```python
from build123d import *

# Parameters (mm, degrees)
BOSS_EXTRUDE1_DEPTH = 25
SKETCH2_R           = 1.5
CUT_EXTRUDE1_DEPTH  = 8
CUT_EXTRUDE2_START  = -8
SKETCH3_R           = 1.5
CUT_EXTRUDE2_DEPTH  = 8


with BuildPart() as part:
    # Sketch1 → Boss-Extrude1 (new, symmetric)
    with BuildSketch(Plane(origin=(0, 0, 0), x_dir=(1, 0, 0), z_dir=(0, 1, 0))):
        Polygon((2.655811238, 0), (1.327905619, 2.3), (-1.327905619, 2.3), (-2.655811238, 0), (-1.327905619, -2.3), (1.327905619, -2.3), align=None)
    extrude(amount=BOSS_EXTRUDE1_DEPTH, both=True)

    # Sketch2 → Cut-Extrude1 (cut)
    with BuildSketch(Plane(origin=(0, 25, 0), x_dir=(1, 0, 0), z_dir=(0, 1, 0))):
        with Locations(Location((0, 0, 0), (0, 0, 270))):
            Circle(SKETCH2_R)
    extrude(amount=-CUT_EXTRUDE1_DEPTH, mode=Mode.SUBTRACT)

    # Sketch3 → Cut-Extrude2 (cut)
    with BuildSketch(Plane.XZ.offset(25).offset(CUT_EXTRUDE2_START)):
        with Locations(Location((0, 0, 0), (0, 0, 90))):
            Circle(SKETCH3_R)
    extrude(amount=CUT_EXTRUDE2_DEPTH, mode=Mode.SUBTRACT)


solid = part.part
```
Model file for the job. Use its own axes, mm. A direction names the side the tool comes from. Round coordinates to 2 decimals unless told otherwise and drop trailing zeros. Order: outer loops, then holes, each group sorted by start corner. A loop starts at its lowest first (then second) coordinate and runs counter-clockwise, first axis right, second up. Notation, with made-up numbers: (10.25, 59) -> (65.25, 59) arc R32 cw to (65.25, 94) -> close; hole circle Ø1 at (17, 53). An arc over 180 degrees is marked (long way). Use one line per item in the form item = value.
Item 1: Drill centre lines: line 1 (X direction, y = 21, z = 0); line 2 (Y direction, x = 0.45, z = -0.3); line 3 (X direction, y = 13, z = -0.6). Where is each one in solid material? Low to high.
Returned:
line_1 = -2.66 to -1.5, 1.5 to 2.66
line_2 = -17 to 17
line_3 = -2.31 to 2.31
Item 2: Flat gauge pins, fed straight in: pin 1 Ø2.5 at (x, z) = (0, 0) entering from +Y; pin 2 Ø0.9 at (x, z) = (0, 0.5) entering from -Y. Where does each tip first touch, or does it go through?
Returned:
pin_1 = 17
pin_2 = -17
Item 3: Tool access for faces 1 (the face through (0, 0, 2.3)), 2 (the face through (0, -17, 0)), 3 (the face through (0.45, 21.06, 1.43)): list every direction of +Z, -Z, +X, -X, +Y, -Y with a clear straight run to the whole face (end or side of a thin tool).
Returned:
face_1 = +Z, +X, -X, +Y, -Y
face_2 = -Y
face_3 = +Y
Item 4: Cut at B-B, the plane x = 0. Write the cut outline in (y, z), and give its area (3 significant figures).
Returned:
outline = (-25, -2.3) -> (25, -2.3) -> (25, -1.5) -> (17, -1.5) -> (17, 1.5) -> (25, 1.5) -> (25, 2.3) -> (-25, 2.3) -> (-25, 1.5) -> (-17, 1.5) -> (-17, -1.5) -> (-25, -1.5) -> close
area = 182 mm^2
Item 5: Pull direction Z, two halves, no side cores. Call faces 4 (the face through (0, 17, 0)), 5 (the face through (2.001, 0.35, -1.134)), 6 (the face through (-2.001, 0.35, 1.134)): released by +Z, released by -Z, zero draft, split by the parting line, or undercut.
Returned:
face_4 = undercut
face_5 = released by -Z
face_6 = released by +Z
Item 6: Cut at D-D, the plane y = -11. Write the cut outline in (x, z), and give its area (3 significant figures).
Returned:
outline = (-2.66, 0) -> (-1.33, -2.3) -> (1.33, -2.3) -> (2.66, 0) -> (1.33, 2.3) -> (-1.33, 2.3) -> close
area = 18.3 mm^2
Item 7: Cut at A-A, the plane y = -19. Write the cut outline in (x, z), and give its area (3 significant figures).
Returned:
outline = (-2.66, 0) -> (-1.33, -2.3) -> (1.33, -2.3) -> (2.66, 0) -> (1.33, 2.3) -> (-1.33, 2.3) -> close; hole circle Ø3 at (0, 0)
area = 11.3 mm^2
Item 8: Cut at C-C, the plane z = 0.85. Write the cut outline in (x, y), and give its area (3 significant figures).
Returned:
outline = (-2.17, -25) -> (-1.24, -25) -> (-1.24, -17) -> (1.24, -17) -> (1.24, -25) -> (2.17, -25) -> (2.17, 25) -> (1.24, 25) -> (1.24, 17) -> (-1.24, 17) -> (-1.24, 25) -> (-2.17, 25) -> close
area = 177 mm^2
